Input: part model. Units: mm. Frame: model coordinates. A direction names the side the tool comes from. Round coordinates to 2 decimals unless told otherwise and drop trailing zeros. Loops run counter-clockwise (first coordinate to the right, second up) from the corner with the lowest first, then second, coordinate; pieces in that order, holes last. Notation, with made-up numbers: (-14.5, -19) - (10.5, -19) arc R25 ccw to (10.5, 18) - close; hole circle Ø11 at (39, 81.25). An arc over 180 degrees is marked (long way). Write each question's results on one line, items separated by ' | '.
from build123d import *

# Parameters (mm, degrees)
RESSALTO_EXTRUS_O1_DEPTH = 4.5


with BuildPart() as part:
    # Esboço1 → Ressalto-extrusão1 (new, symmetric)
    with BuildSketch(Plane.XY):
        with BuildLine():
            ThreePointArc((91.591504601, -7.191966904), (97.92602, 0), (91.591504601, 7.191966904))
            Line((91.591504601, 7.191966904), (2.361318902, 18.550314635))
            ThreePointArc((2.361318902, 18.550314635), (-18.7, 0), (2.361318902, -18.550314635))
            Line((2.361318902, -18.550314635), (91.591504601, -7.191966904))
        make_face()
        with BuildLine():
            ThreePointArc((1.982497688, -15.57432833), (-15.7, 0), (1.982497688, 15.57432833))
            Line((1.982497688, 15.57432833), (91.212683387, 4.215980599))
            ThreePointArc((91.212683387, 4.215980599), (94.92602, 0), (91.212683387, -4.215980599))
            Line((91.212683387, -4.215980599), (1.982497688, -15.57432833))
        make_face(mode=Mode.SUBTRACT)
    extrude(amount=RESSALTO_EXTRUS_O1_DEPTH, both=True)


solid = part.part
1. Set-up query: faces 1 (the flat face through (47.6, 12.79, 0.06)), 2 (the cylindrical face through (94.925, 0.086, 0.063)). Return all of +Z, -Z, +X, -X, +Y, -Y with unobstructed straight access to the full face (end or side cutting, diameter ignored); none if empty.
Answer:
face 1: +Z, -Z, +X, +Y | face 2: +Z, -Z
2. Line query: line 1 (Y direction, x = 0, z = -1); line 2 (Y direction, x = 45, z = 3.25); line 3 (X direction, y = -1.5, z = 2.5). Output: solid intervals per line, ascending. Write a range as [from, to].
Answer:
line 1: [-18.7, -15.7], [15.7, 18.7] | line 2: [-13.12, -10.1], [10.1, 13.12] | line 3: [-18.64, -15.63], [94.65, 97.77]
3. Mould query, pull axis X, two halves, no side actions, for faces 3 (the flat face through (39.3, 11.2, -4.5)), 4 (the cylindrical face through (97.925, -0.147, 0.063)), 5 (the flat face through (47.222, -9.816, 0.063)). Classes: pulls with the +X half, pulls with the -X half, needs draft (parallel to the pull), parting line crosses it, or undercut.
Answer:
face 3: needs draft | face 4: pulls with the +X half | face 5: undercut
4. Section query C-C, the plane x = -7.5. Output: boundary loops of the cut face in (y, z), plus the area to 3 significant figures.
Answer:
outline: (-17.13, -4.5) - (-13.79, -4.5) - (-13.79, 4.5) - (-17.13, 4.5) - close; (13.79, -4.5) - (17.13, -4.5) - (17.13, 4.5) - (13.79, 4.5) - close | area: 60.1 mm^2
5. Section query B-B, the plane z = 3.5. Output: boundary loops of the cut face in (x, y).
Answer:
outline: (2.36, -18.55) - (91.59, -7.19) arc R7.25 ccw to (91.59, 7.19) - (2.36, 18.55) arc R18.7 ccw (long way) to start; hole (1.98, -15.57) - (91.21, -4.22) arc R4.25 ccw to (91.21, 4.22) - (1.98, 15.57) arc R15.7 ccw (long way) to start
6. Section query A-A, the plane y = 0. Output: boundary loops of the cut face in (x, z), plus the area to 3 significant figures.
Answer:
outline: (-18.7, -4.5) - (-15.7, -4.5) - (-15.7, 4.5) - (-18.7, 4.5) - close; (94.93, -4.5) - (97.93, -4.5) - (97.93, 4.5) - (94.93, 4.5) - close | area: 54.0 mm^2
7. Contact query for flat-ended pins moving along their axis: pin 1 (1.5 mm diameter, centred on x = 83.5, z = -1, fed in from -Y); pin 2 (4 mm diameter, centred on x = 56.5, z = 2.5, fed in from +Y); pin 3 (5 mm diameter, centred on x = 14.5, z = 3, fed in from -Y). Output: stop coordinate, or through.
Answer:
pin 1: y = -8.32 | pin 2: y = 11.91 | pin 3: y = -17.32
